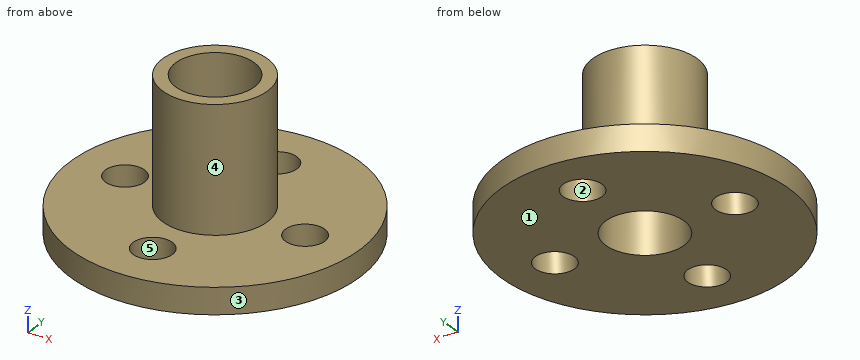
from build123d import *

# Parameters (mm, degrees)
SKETCH_2_R          = 1.5
CUT_EXTRUDE_1_DEPTH = 10


with BuildPart() as part:
    # 草图1 → 旋转1 (revolve)
    with BuildSketch(Plane(origin=(0, 0, 0), x_dir=(1, 0, 0), z_dir=(0, 1, 0))):
        Polygon((0, 0), (-8, 0), (-8, -2), (-1, -2), (-1, -11.5), (0, -11.5), align=None)
    revolve(axis=Axis((3, 0, -3.355756156), (0, 0, 1)))

    # 草图2 → 切除-拉伸1 (cut)
    with BuildSketch(Plane(origin=(0, 0, 0), x_dir=(-1, 0, 0), z_dir=(0, 0, -1))):
        with Locations((-3, 7)):
            Circle(SKETCH_2_R)
        with Locations((4, 0)):
            Circle(SKETCH_2_R)
        with Locations((-3, -7)):
            Circle(SKETCH_2_R)
        with Locations((-10, 0)):
            Circle(SKETCH_2_R)
    extrude(amount=-CUT_EXTRUDE_1_DEPTH, mode=Mode.SUBTRACT)


solid = part.part
The listing builds one solid part. Answer for the finished solid, in the listing's coordinates (mm). Face numbers are marked on the shaded views. A direction names the side the tool comes from. Give positions to 0.01 mm unless a question says otherwise; leave off trailing zeros. Order: outer loops, then holes, each group sorted by start corner. A loop starts at its lowest first (then second) coordinate and runs counter-clockwise, first axis right, second up. Notation, with made-up numbers: (75.25, 34) - (80.25, 34) arc R31 cw to (80.25, 62) - close; hole circle Ø11 at (16.5, 53.5). An arc over 180 degrees is marked (long way). Use one line per item in the form item = value.
1) Find section D-D on z = 7. Determine the outline of the cut face in (x, y), and give its area (3 significant figures).
Verdict:
outline = circle Ø8 at (3, 0); hole circle Ø6 at (3, 0)
area = 22.0 mm^2
2) Find section B-B on y = 0. Determine the outline of the cut face in (x, z), and give its area (3 significant figures).
Verdict:
outline = (-8, 0) - (-5.5, 0) - (-5.5, 2) - (-8, 2) - close; (-2.5, 0) - (0, 0) - (0, 11.5) - (-1, 11.5) - (-1, 2) - (-2.5, 2) - close; (6, 0) - (8.5, 0) - (8.5, 2) - (7, 2) - (7, 11.5) - (6, 11.5) - close; (11.5, 0) - (14, 0) - (14, 2) - (11.5, 2) - close
area = 39.0 mm^2
3) Consider probe 1 along Y at (x, z) = (3, 1); probe 2 along X at (y, z) = (0, 8); probe 3 along X at (y, z) = (1.25, 1). Determine where each line is inside the solid, lowest interval first. Write a range as [from, to].
Verdict:
probe_1 = [-11, -8.5], [-5.5, -3], [3, 5.5], [8.5, 11]
probe_2 = [-1, 0], [6, 7]
probe_3 = [-7.93, -4.83], [-3.17, 0.27], [5.73, 9.17], [10.83, 13.93]
4) The mould has two halves that part along Y. Classify the marked faces 1, 2 and 3: released by +Y, released by -Y, zero draft, split by the parting line, or undercut.
Verdict:
face_1 = zero draft
face_2 = undercut
face_3 = split by the parting line
5) For the marked faces 4 and 5, determine the directions among +Z, -Z, +X, -X, +Y, -Y from which every point of the face is accessible in a straight line to the end or side of a thin tool.
Verdict:
face_4 = +Z
face_5 = +Z, -Z
6) Find section A-A on x = 3. Determine the outline of the cut face in (y, z), and give its area (3 significant figures).
Verdict:
outline = (-11, 0) - (-8.5, 0) - (-8.5, 2) - (-11, 2) - close; (-5.5, 0) - (-3, 0) - (-3, 11.5) - (-4, 11.5) - (-4, 2) - (-5.5, 2) - close; (3, 0) - (5.5, 0) - (5.5, 2) - (4, 2) - (4, 11.5) - (3, 11.5) - close; (8.5, 0) - (11, 0) - (11, 2) - (8.5, 2) - close
area = 39.0 mm^2
7) Find section C-C on y = -7. Determine the outline of the cut face in (x, z), and give its area (3 significant figures).
Verdict:
outline = (-5.49, 0) - (1.5, 0) - (1.5, 2) - (-5.49, 2) - close; (4.5, 0) - (11.49, 0) - (11.49, 2) - (4.5, 2) - close
area = 27.9 mm^2
8) Each of these flat-tipped pins is pushed along its axis until it touches: pin 1 (6 mm diameter, centred on y = 0, z = 7.5, fed in from -X); pin 2 (1 mm diameter, centred on x = 3, y = -5, fed in from +Z); pin 3 (2.5 mm diameter, centred on x = 3, y = -7, fed in from -Z); pin 4 (3 mm diameter, centred on y = -2.5, z = 2, fed in from -X). Where does it stop, or does it pass through?
Verdict:
pin_1 = -1
pin_2 = 2
pin_3 = through
pin_4 = -7.95
